Could you check a few things on this drawing? It's one solid part, dimensions in mm from its lowest x, y, z. A direction names the side the tool comes from. Give positions to 0.01 mm unless a question says otherwise; leave off trailing zeros. Loops run counter-clockwise (first coordinate to the right, second up) from the corner with the lowest first, then second, coordinate; pieces in that order, holes last. Notation, with made-up numbers: M -15,48 L 24,48 A27 ccw 24,72 Z; hole C 41,-6.75 d5. An arc over 180 degrees is marked long. Return JSON: item names as keys, results as strings. Group by question number.
1. If we section it at A-A (y = 12.5): Write out the boundary of the cut face in (x, z), plus the area to 4 significant figures.
2. If we section it at D-D (z = 13.5): Write out the boundary of the cut face in (x, y).
3. If we mould it in two halves opening along X, with no side actions, what happens to the marked faces 1, 2 and 3? For each: +X half, -X half, draft (parallel to the pull), parting line (faces both ways), or undercut.
4. For the marked faces 4 and 5, which set-ups out of +Z, -Z, +X, -X, +Y, -Y let a thin tool reach every point of the face, with its end or its side?
5. For pin 1 (3 mm diameter, centred on x = 18, z = 11, fed in from +Y); pin 2 (7.5 mm diameter, centred on x = 29.5, y = 12.5, fed in from -Z), each with a flat end and sliding along its axis, tell me the tip position at first contact or that it passes through.
6. Please list where these lines run through material, in increasing order: line 1 (Y direction, x = 37, z = 27); line 2 (Z direction, x = 39, y = 8); line 3 (X direction, y = 11.5, z = 27).
7. If we section it at C-C (x = 20): Write out the boundary of the cut face in (y, z).
8. If we section it at B-B (x = 37): Write out the boundary of the cut face in (y, z).
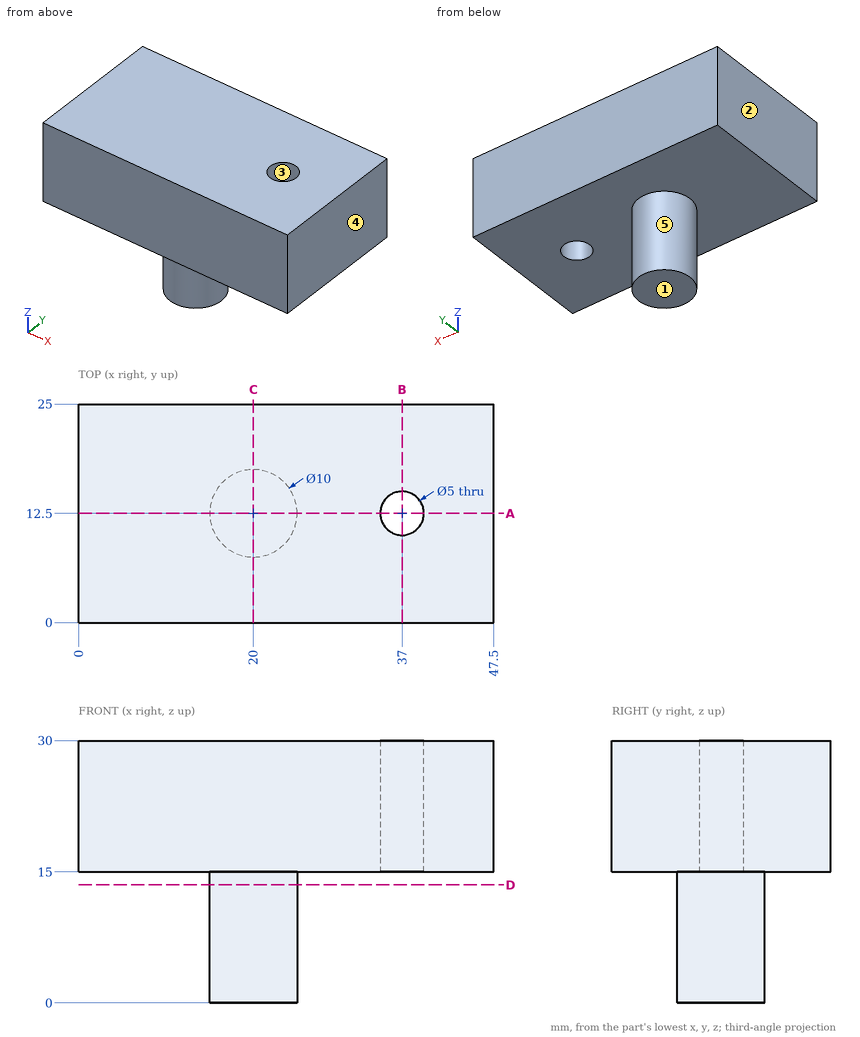
Answer:
{
 "1": {"outline": "M 0,15 L 15,15 L 15,0 L 25,0 L 25,15 L 34.5,15 L 34.5,30 L 0,30 Z; M 39.5,15 L 47.5,15 L 47.5,30 L 39.5,30 Z", "area": "787.5 mm²"},
 "2": {"outline": "C 20,12.5 d10"},
 "3": {"face 1": "draft", "face 2": "-X half", "face 3": "undercut"},
 "4": {"face 4": "+Z, -Z, +X, +Y, -Y", "face 5": "-Z"},
 "5": {"pin 1": "stops at y = 17.47", "pin 2": "stops at z = 15"},
 "6": {"line 1": "y = 0 to 10, 15 to 25", "line 2": "z = 15 to 30", "line 3": "x = 0 to 34.71, 39.29 to 47.5"},
 "7": {"outline": "M 0,15 L 7.5,15 L 7.5,0 L 17.5,0 L 17.5,15 L 25,15 L 25,30 L 0,30 Z"},
 "8": {"outline": "M 0,15 L 10,15 L 10,30 L 0,30 Z; M 15,15 L 25,15 L 25,30 L 15,30 Z"}
}
